from build123d import *

# Parameters (mm, degrees)
F0_R          = 2.5
F0_W          = 44.5
F0_H          = 1
F0_W_2        = 1
F0_H_2        = 32
F1_DEPTH      = 13
F2_R          = 7.5
F3_DEPTH      = 50
F4_R          = 12.99999
F2_W          = 3
F2_H          = 8
F5_DEPTH      = 50
F6_DEPTH      = 50
F6_DEPTH_BACK = 25


# Not quite as in the source:
# - a fillet or chamfer is up to 0.001 mm smaller than in the source, because OpenCascade refuses the exact size
# - a feature names something its author has since deleted; it is built from what else it names


with BuildPart() as f1:
    # F0 (on Top) → F1 (new body, symmetric)
    with BuildSketch(Plane.XY):
        Polygon((50, 45), (50, 65), (-40, 65), (-50, 65), (-50, -45), (-40, -45), (50, -45), (50, -34.6913893335), (50, 40), align=None)
        with Locations((-40, -40)):
            Circle(F0_R, mode=Mode.SUBTRACT)
        with Locations((40, -40)):
            Circle(F0_R, mode=Mode.SUBTRACT)
        with Locations((-40, 40)):
            Circle(F0_R, mode=Mode.SUBTRACT)
        Polygon((0.5, 32.5), (45, 32.5), (45, 0.5), (45, -0.5), (45, -32.5), (0.5, -32.5), (-0.5, -32.5), (-45, -32.5), (-45, -0.5), (-45, 0.5), (-45, 32.5), (-0.5, 32.5), align=None, mode=Mode.SUBTRACT)
        with Locations((40, 40)):
            Circle(F0_R, mode=Mode.SUBTRACT)
        Polygon((-40, -45), (-50, -45), (-50, -65), (50, -65), (50, -45), align=None)
        with Locations((22.75, 0)):
            Rectangle(F0_W, F0_H)
        with Locations((-22.75, 0)):
            Rectangle(F0_W, F0_H)
        Rectangle(F0_W_2, F0_H)
        with Locations((0, -16.5)):
            Rectangle(F0_W_2, F0_H_2)
        with Locations((0, 16.5)):
            Rectangle(F0_W_2, F0_H_2)
    extrude(amount=F1_DEPTH, both=True)

    # F2 (on Right) → F3 (cut, symmetric)
    with BuildSketch(Plane.YZ):
        with Locations((54.5, 0)):
            Circle(F2_R)
        with Locations((-54.5, 0)):
            Circle(F2_R)
    extrude(amount=F3_DEPTH, both=True, mode=Mode.SUBTRACT)

    # F4 (radius 13 in the source; OpenCascade refuses exactly that, so slightly less here)
    f4_edges = [f1.edges().sort_by_distance(p)[0] for p in [
        (0, 65, 13),
        (0, 65, -13),
        (0, -65, 13),
        (0, -65, -13),
    ]]
    fillet(f4_edges, radius=F4_R)

    # F2 (on Right) → F5 (cut)
    with BuildSketch(Plane.YZ):
        with Locations((-18.3, -4)):
            Rectangle(F2_W, F2_H)
        with Locations((-12.3, -4)):
            Rectangle(F2_W, F2_H)
        with Locations((12.3, 4)):
            Rectangle(F2_W, F2_H)
        with Locations((18.3, 4)):
            Rectangle(F2_W, F2_H)
    extrude(amount=-F5_DEPTH, mode=Mode.SUBTRACT)

    # F2 (on Right) → F6 (cut, two sides)
    with BuildSketch(Plane.YZ) as f6_sk:
        with Locations((12.3, -4)):
            Rectangle(F2_W, F2_H)
        with Locations((18.3, -4)):
            Rectangle(F2_W, F2_H)
        with Locations((-12.3, 4)):
            Rectangle(F2_W, F2_H)
        with Locations((-18.3, 4)):
            Rectangle(F2_W, F2_H)
    extrude(amount=F6_DEPTH, mode=Mode.SUBTRACT)
    extrude(f6_sk.sketch, amount=-F6_DEPTH_BACK, mode=Mode.SUBTRACT)


solid = f1.part
Can you work these out from the model? Positions are in its coordinate system, mm. A direction names the side the tool comes from. Coordinates: 2 decimals unless noted, no trailing zeros. Order: outer loops, then holes, each group sorted by start corner. A loop starts at its lowest first (then second) coordinate and runs counter-clockwise, first axis right, second up. Notation, with made-up numbers: (-6.5, 44) - (5.5, 44) arc R15 ccw to (5.5, 48) - close; hole circle Ø7 at (-10.75, 81). An arc over 180 degrees is marked (long way). Answer as a JSON object with one key per item and string values. Group by question number.
Q1. On a 3-axis mill with a long thin cutter (end or side, diameter ignored), from which of +Z, -Z, +X, -X, +Y, -Y can I reach the whole of each face in a straight line? I mean faces 4 (the face through (-47, -12, 0)), 5 (the face through (-23, -0.5, 0)), 6 (the face through (47, 10.8, -4)). Say none if no direction works.
Q2. Imagine slicing it at B-B (y = 24.5). Please give me the cut outline in (x, z).
Q3. I need wall thicknesses on line 1 (X direction, y = 2.5, z = 11.5); line 2 (Y direction, x = -13, z = 2.25); line 3 (Y direction, x = 6.5, z = 8). Which ranges of each line are inside material? Lowest first, please. Write a range as from..to.
Q4. We'd pull the mould along X, two halves only. Please class faces 1 (the face through (47, -19.8, 4)), 2 (the face through (23, -32.5, 0)), 3 (the face through (50, -1, 0)): +X half, -X half, draft (parallel to the pull), parting line (faces both ways), or undercut.
Q5. Will these pins go through, and if not, where does the flat tip stop? P1, Ø0.6, axis at x = 0, z = -6, coming from the -Y side; P2, Ø1.5, axis at x = -38, z = -7.5, coming from the +Y side; P3, Ø4, axis at x = -7, z = 7.5, coming from the +Y side.
Q6. Imagine slicing it at A-A (x = 4). Give the number of separate pieces and of enclosed holes in the cut face, and give its area (3 significant figures).
Determined:
{
 "1": {"face 4": "-X", "face 5": "+Z, -Z", "face 6": "+X"},
 "2": {"outline": "(-50, -13) - (-45, -13) - (-45, 13) - (-50, 13) - close; (-0.5, -13) - (0.5, -13) - (0.5, 13) - (-0.5, 13) - close; (45, -13) - (50, -13) - (50, 13) - (45, 13) - close"},
 "3": {"line 1": "x = -50..-45, -0.5..0.5, 45..50", "line 2": "y = -64.8..-61.65, -47.35..-32.5, -0.5..0.5, 32.5..47.35, 61.65..64.8", "line 3": "y = -62.25..-32.5, -0.5..0.5, 32.5..62.25"},
 "4": {"face 1": "draft", "face 2": "undercut", "face 3": "+X half"},
 "5": {"P1": "stops at y = -63.68", "P2": "stops at y = 63.11", "P3": "stops at y = 63.78"},
 "6": {"separate pieces": "3", "enclosed holes": "2", "area": "1,220 mm2"}
}
